Input: part model. Units: mm. Frame: model coordinates. A direction names the side the tool comes from. Give positions to 0.01 mm unless a question says otherwise; leave off trailing zeros. Write each loop counter-clockwise with the first axis right and the second up, starting at its lowest first coordinate (ties: lowest second). Pieces come first, ordered by that corner, then holes. Notation, with made-up numbers: (26, -37) -> (30, -37) arc R30 cw to (30, -15) -> close; hole circle Ø2 at (-24.75, 23.25). An arc over 180 degrees is marked (long way). Return JSON: item names as keys, results as strings. Group by question number.
Item 1: Section D-D, the plane x = 4. Return loops of the section in (y, z).
Item 2: Section B-B, the plane y = 3. Return loops of the section in (x, z).
Item 3: Line query: line 1 (Y direction, x = 0, z = 2.4); line 2 (Y direction, x = 35, z = 2.05); line 3 (Z direction, x = 10.5, y = 1). Output: solid intervals per line, ascending. Write a range as [from, to].
Item 4: Mould query, pull axis Y, two halves, no side actions, for faces 4 (the face through (38, -10, 1)), 5 (the face through (50, 0, 0)), 6 (the face through (25, 17.5, 2)). Classes: released by +Y, released by -Y, zero draft, split by the parting line, or undercut.
Item 5: Section C-C, the plane z = -0.65. Return loops of the section in (x, y), then the cut area to 3 significant figures.
Item 6: Pin query (flat end, axial travel): P1, Ø2, axis at x = 4.5, z = -1.5, coming from the -Y side; P2, Ø1.5, axis at y = 7.5, z = -1.5, coming from the -X side; P3, Ø3.5, axis at y = 10.5, z = 1, coming from the -X side; P4, Ø4, axis at x = 36.375, y = 0, coming from the +Z side. Return the tip coordinate at first contact, or that it passes through.
Item 7: Set-up query: faces 1 (the face through (15, 0, 0)), 2 (the face through (17, 0, 3)), 3 (the face through (36.411, -4.875, 1.479)). Return all of +Z, -Z, +X, -X, +Y, -Y with unobstructed straight access to the full face (end or side cutting, diameter ignored); none if empty.
Item 8: Section A-A, the plane x = 36. Return loops of the section in (y, z).
from build123d import *

# Parameters (mm, degrees)
SKETCH_1_R      = 1.65
EXTRUDE_1_DEPTH = 3
SKETCH_2_W      = 3
SKETCH_2_H      = 35
EXTRUDE_2_DEPTH = 6


with BuildPart() as part:
    # 草图1 → 凸台-拉伸1 (new body)
    with BuildSketch(Plane.XY):
        with BuildLine():
            Line((0, 17.5), (50, 17.5))
            Line((50, 17.5), (50, -17.5))
            Line((50, -17.5), (0, -17.5))
            ThreePointArc((0, -17.5), (-17.5, 0), (0, 17.5))
        make_face()
        with Locations((36.375, 0)):
            Circle(SKETCH_1_R, mode=Mode.SUBTRACT)
        with Locations((0, 6)):
            Circle(SKETCH_1_R, mode=Mode.SUBTRACT)
        with Locations((0, -6)):
            Circle(SKETCH_1_R, mode=Mode.SUBTRACT)
        with BuildLine():
            Line((34.75, 12.5), (34.75, 6.5))
            ThreePointArc((34.75, 6.5), (36.375, 4.875), (38, 6.5))
            Line((38, 6.5), (38, 12.5))
            ThreePointArc((38, 12.5), (36.375, 14.125), (34.75, 12.5))
        make_face(mode=Mode.SUBTRACT)
        with BuildLine():
            Line((34.75, -6.5), (34.75, -12.5))
            ThreePointArc((34.75, -12.5), (36.375, -14.125), (38, -12.5))
            Line((38, -12.5), (38, -6.5))
            ThreePointArc((38, -6.5), (36.375, -4.875), (34.75, -6.5))
        make_face(mode=Mode.SUBTRACT)
    extrude(amount=EXTRUDE_1_DEPTH)

    # 草图2 → 凸台-拉伸2 (add)
    with BuildSketch(Plane.XY.offset(3)):
        with Locations((48.5, 0)):
            Rectangle(SKETCH_2_W, SKETCH_2_H)
    extrude(amount=-EXTRUDE_2_DEPTH)


solid = part.part
Answer below:
{
 "1": {"outline": "(-17.5, 0) -> (17.5, 0) -> (17.5, 3) -> (-17.5, 3) -> close"},
 "2": {"outline": "(-17.24, 0) -> (47, 0) -> (47, -3) -> (50, -3) -> (50, 3) -> (-17.24, 3) -> close"},
 "3": {"line 1": "y = [-17.5, -7.65], [-4.35, 4.35], [7.65, 17.5]", "line 2": "y = [-17.5, -13.37], [-5.63, -0.91], [0.91, 5.63], [13.37, 17.5]", "line 3": "z = [0, 3]"},
 "4": {"face 4": "undercut", "face 5": "zero draft", "face 6": "released by +Y"},
 "5": {"outline": "(47, -17.5) -> (50, -17.5) -> (50, 17.5) -> (47, 17.5) -> close", "area": "105 mm2"},
 "6": {"P1": "passes through", "P2": "stops at x = 47", "P3": "stops at x = -15.16", "P4": "stops at z = 3"},
 "7": {"face 1": "-Z, -X, +Y, -Y", "face 2": "+Z, +X, -X, +Y, -Y", "face 3": "+Z, -Z"},
 "8": {"outline": "(-17.5, 0) -> (-14.08, 0) -> (-14.08, 3) -> (-17.5, 3) -> close; (-4.92, 0) -> (-1.61, 0) -> (-1.61, 3) -> (-4.92, 3) -> close; (1.61, 0) -> (4.92, 0) -> (4.92, 3) -> (1.61, 3) -> close; (14.08, 0) -> (17.5, 0) -> (17.5, 3) -> (14.08, 3) -> close"}
}
